from build123d import *

# Parameters (mm, degrees)
SKETCH2_R           = 3.1
BOSS_EXTRUDE2_DEPTH = 6


with BuildPart() as part:
    # Sketch2 → Boss-Extrude2 (new body)
    with BuildSketch(Plane.XY):
        with BuildLine():
            Line((100, -56), (-105, -56))
            add(Edge.make_bspline(
                [(-170.77007734, 39.000109259), (-170.755319597, 38.457683604), (-170.706798384, 36.537887441), (-170.637287988, 33.122957729), (-170.5261489, 27.184054493), (-170.34340093, 19.366986891), (-169.889474506, 9.608710222), (-169.039164203, -0.266842999), (-167.1706255, -13.234272429), (-163.891886546, -25.351425111), (-158.719183516, -35.536226847), (-153.788973421, -41.996369681), (-147.740986476, -47.090640281), (-140.115988759, -50.864892697), (-131.329474875, -53.495779888), (-123.622789186, -54.830760959), (-117.546310091, -55.488589317), (-113.112089799, -55.803916745), (-109.593584136, -55.942092458), (-106.905885897, -55.99243235), (-105.641968688, -55.999999365), (-105, -56)],
                knots=[0.050003059, 0.050003059, 0.050003059, 0.050003059, 0.0625, 0.09375, 0.125, 0.1875, 0.25, 0.3125, 0.375, 0.5, 0.5625, 0.625, 0.6875, 0.75, 0.8125, 0.875, 0.90625, 0.9375, 0.96875, 0.984375, 1, 1, 1, 1], degree=3))
            Line((-170.77007734, 39.000109259), (-170.770080313, 51))
            Line((-170.770080313, 51), (159.005500018, 51))
            Line((159.005500018, 51), (170.770080313, 51))
            Line((170.770080313, 51), (170.770074367, 39.000109259))
            add(Edge.make_bspline(
                [(105, -56), (105.641968688, -55.999999365), (106.905885897, -55.99243235), (109.593584136, -55.942092457), (113.112089799, -55.803916745), (117.546310092, -55.488589317), (123.622789186, -54.830760959), (131.329474876, -53.495779888), (140.11598876, -50.864892696), (147.740986477, -47.09064028), (153.788973422, -41.996369679), (158.719183518, -35.536226846), (163.891886547, -25.351425109), (167.170625501, -13.234272427), (169.039164203, -0.266842997), (169.889474507, 9.608710225), (170.343400931, 19.366986894), (170.5261489, 27.184054497), (170.637287988, 33.122957733), (170.706798384, 36.537887444), (170.755319597, 38.457683605), (170.770074367, 39.000109259)],
                knots=[0, 0, 0, 0, 0.015625, 0.03125, 0.0625, 0.09375, 0.125, 0.1875, 0.25, 0.3125, 0.375, 0.4375, 0.5, 0.625, 0.6875, 0.75, 0.8125, 0.875, 0.90625, 0.9375, 0.949996941, 0.949996941, 0.949996941, 0.949996941], degree=3))
            Line((105, -56), (100, -56))
        make_face()
        with Locations((164.770080313, 32.55449126)):
            Circle(SKETCH2_R, mode=Mode.SUBTRACT)
        with Locations((-156.770064318, -13.565854924)):
            Circle(SKETCH2_R, mode=Mode.SUBTRACT)
        with Locations((-164.770080313, 32.55449126)):
            Circle(SKETCH2_R, mode=Mode.SUBTRACT)
        with Locations((156.770064318, -13.565854924)):
            Circle(SKETCH2_R, mode=Mode.SUBTRACT)
    extrude(amount=BOSS_EXTRUDE2_DEPTH)


solid = part.part
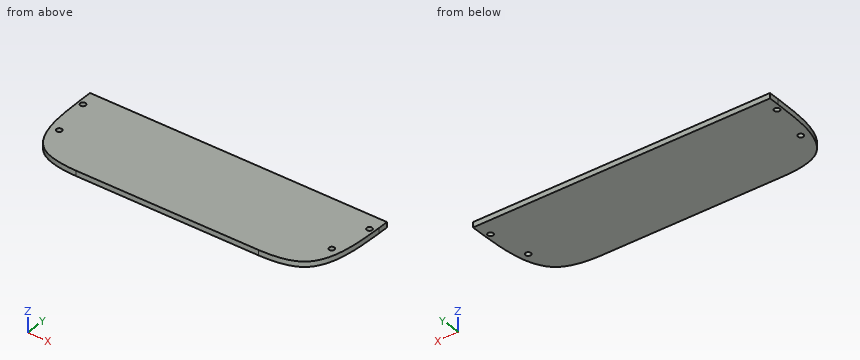
Can you work these out from the model? Positions are in its coordinate system, mm. Give positions to 0.01 mm unless a question says otherwise; leave off trailing zeros. Write each question's results on one line, items separated by ' | '.
1) Suppose I cut it at A-A, the plane z = 3. Give the number of separate pieces and of enclosed holes in the cut face, then the cut area to 3 significant figures.
Final values:
separate pieces: 1 | enclosed holes: 4 | area: 34,900 mm^2
2) Please list where these lines run through material, in increasing order: line 1 along X through (y, z) = (30.5, 2); line 2 along X through (y, z) = (36.5, 4); line 3 along X through (y, z) = (5, 5). Write a range as [from, to].
Final values:
line 1: x = [-170.59, -167.09], [-162.45, 162.45], [167.09, 170.59] | line 2: x = [-170.71, 170.71] | line 3: x = [-169.47, 169.47]
3) I'm going to push flat-ended pins straight in: pin 1 Ø1.5 at (y, z) = (-34.5, 2) entering from -X; pin 2 Ø8 at (x, y) = (164.77, 32.55) entering from -Z. Where does each tip first touch, or does it pass through?
Final values:
pin 1: stops at x = -159.49 | pin 2: stops at z = 0
